The model under review builds one solid part; all positions refer to its coordinate system, in mm. A direction names the side the tool comes from. Give positions to 0.01 mm unless a question says otherwise; leave off trailing zeros. Loops run counter-clockwise (first coordinate to the right, second up) from the corner with the lowest first, then second, coordinate; pieces in that order, holes last. Notation, with made-up numbers: (-27.75, 13) - (-19.75, 13) arc R17 cw to (-19.75, 37) - close; hole circle Ø5 at (74.25, 8.5). An arc over 180 degrees is marked (long way). Return JSON: item names as keys, results as strings. Group by question number.
```python
from build123d import *

# Parameters (mm, degrees)
BOSS_EXTRUDE1_DEPTH = 4.5
DIAMETER_HOLE1_D    = 4.5
CHAMFER1_SIZE       = 2
SKETCH4_R           = 2
CUT_EXTRUDE1_DEPTH  = 30.757352033


with BuildPart() as part:
    # Sketch1 → Boss-Extrude1 (new, symmetric)
    with BuildSketch(Plane.XY):
        Polygon((12.5, 0), (-12.5, 0), (-12.5, 5), (-3, 5), (-3, 25), (3, 25), (3, 5), (12.5, 5), align=None)
    extrude(amount=BOSS_EXTRUDE1_DEPTH, both=True)

    # Diameter Hole1 (through all)
    with Locations(Plane(origin=(0, 5, 0), x_dir=(1, 0, 0), z_dir=(0, 1, 0))):
        with Locations((-8.5, 0), (8.5, 0)):
            Hole(DIAMETER_HOLE1_D / 2)

    # Chamfer1
    chamfer1_edges = [part.edges().sort_by_distance(p)[0] for p in [
        (0, 25, 4.5),
        (0, 25, -4.5),
    ]]
    chamfer(chamfer1_edges, length=CHAMFER1_SIZE)

    # Sketch4 → Cut-Extrude1 (cut, through all)
    with BuildSketch(Plane(origin=(3, 0, 0), x_dir=(0, 0, -1), z_dir=(1, 0, 0))):
        with Locations(Location((0, 20, 0), (0, 0, 90))):
            Circle(SKETCH4_R)
    extrude(amount=-CUT_EXTRUDE1_DEPTH, mode=Mode.SUBTRACT)


solid = part.part
```
1) To check wall thickness, follow line 1 (Z direction, x = -8.5, y = 2); line 2 (Z direction, x = -0.75, y = 20); line 3 (Y direction, x = 9.75, z = -3.75). State the ranges of each line that lie inside material, in increasing order.
2) We need section C-C, the plane x = 8.5. Write out the cut boundary in (y, z), plus the area to 3 significant figures.
3) For pin 1 Ø4.5 at (x, z) = (8, -1.5) entering from +Y; pin 2 Ø1 at (x, z) = (7, -0.5) entering from +Y; pin 3 Ø5 at (y, z) = (20, 0) entering from -X, all flat-tipped, find the tip position at first contact; note any pin that passes through.
4) We need section D-D, the plane y = 19.5. Write out the cut boundary in (x, z).
5) Tool access review of faces 1 (the face through (-3, 15, 0)), 2 (the face through (6, 5, 0)), 3 (the face through (12.5, 3, 0)): name each direction out of +Z, -Z, +X, -X, +Y, -Y from which nothing blocks a thin tool from reaching the whole face with its end or side.
6) Draft analysis for pull direction Z (two halves, no side actions). For faces 4 (the face through (10.748, 2.465, -0.099)), 5 (the face through (0, 9, 4.5)), 6 (the face through (3, 15, 0)), state which applies: +Z half, -Z half, draft (parallel to the pull), parting line (faces both ways), or undercut.
7) We need section B-B, the plane y = 3.5. Write out the cut boundary in (x, z), plus the area to 3 significant figures.
8) We need section A-A, the plane z = 0. Write out the cut boundary in (x, y), plus the area to 3 significant figures.
Findings:
{
 "1": {"line 1": "z = -4.5 to -2.25, 2.25 to 4.5", "line 2": "z = -4.5 to -2, 2 to 4.5", "line 3": "y = 0 to 5"},
 "2": {"outline": "(0, -4.5) - (5, -4.5) - (5, -2.25) - (0, -2.25) - close; (0, 2.25) - (5, 2.25) - (5, 4.5) - (0, 4.5) - close", "area": "22.5 mm^2"},
 "3": {"pin 1": "stops at y = 5", "pin 2": "passes through", "pin 3": "stops at x = -3"},
 "4": {"outline": "(-3, -4.5) - (3, -4.5) - (3, -1.94) - (-3, -1.94) - close; (-3, 1.94) - (3, 1.94) - (3, 4.5) - (-3, 4.5) - close"},
 "5": {"face 1": "+Z, -Z, -X, +Y", "face 2": "+Z, -Z, +X, +Y", "face 3": "+Z, -Z, +X, +Y, -Y"},
 "6": {"face 4": "undercut", "face 5": "+Z half", "face 6": "draft"},
 "7": {"outline": "(-12.5, -4.5) - (12.5, -4.5) - (12.5, 4.5) - (-12.5, 4.5) - close; hole circle Ø4.5 at (-8.5, 0); hole circle Ø4.5 at (8.5, 0)", "area": "193 mm^2"},
 "8": {"outline": "(-12.5, 0) - (-10.75, 0) - (-10.75, 5) - (-12.5, 5) - close; (-6.25, 0) - (6.25, 0) - (6.25, 5) - (3, 5) - (3, 18) - (-3, 18) - (-3, 5) - (-6.25, 5) - close; (-3, 22) - (3, 22) - (3, 25) - (-3, 25) - close; (10.75, 0) - (12.5, 0) - (12.5, 5) - (10.75, 5) - close", "area": "176 mm^2"}
}
